from build123d import *

# Parameters (mm, degrees)
SKETCH002_W     = 13
SKETCH002_H     = 14
SKETCH002_W_2   = 6
PAD001_DEPTH    = 2
SKETCH_R        = 1.6
PAD_DEPTH       = 5
POCKET_DEPTH    = 10.001
SKETCH003_W     = 7
SKETCH003_H     = 5
POCKET001_DEPTH = 17.2330508076
SKETCH004_R     = 1
POCKET002_DEPTH = 6
POCKET003_DEPTH = 3
FILLET_R        = 8
FILLET001_R     = 1
FILLET002_R     = 1


with BuildPart() as pad001:
    # Sketch002 → Pad001 (new body, symmetric)
    with BuildSketch(Plane.XY):
        with Locations((-0.5, 0)):
            Rectangle(SKETCH002_W, SKETCH002_H)
        with Locations((-13, 0)):
            Rectangle(SKETCH002_W_2, SKETCH002_H)
    extrude(amount=PAD001_DEPTH, both=True)


with BuildPart() as fillet002:
    # Sketch → Pad (new body, symmetric)
    with BuildSketch(Plane.XY):
        with BuildLine():
            ThreePointArc((0, -4), (3.9731206567, -0.4629387079), (0.9196556715, 3.8928438764))
            Line((0.9196556715, 3.8928438764), (-8, 6))
            Line((-8, 6), (-30, 6))
            Line((-30, -4), (-30, 6))
            Line((0, -4), (-30, -4))
        make_face()
        Circle(SKETCH_R, mode=Mode.SUBTRACT)
    extrude(amount=PAD_DEPTH, both=True)

    # Sketch001 → Pocket (cut, through all)
    with BuildSketch(Plane(origin=(0, 6, 0), x_dir=(-1, 0, 0), z_dir=(0, 1, 0))):
        Polygon((22, 0.1132486541), (24, -3.3508529611), (24, -5), (30, -5), (30, 5), (27, 5), (27, 3), align=None)
    extrude(amount=-POCKET_DEPTH, mode=Mode.SUBTRACT)

    # Cut: cut Pad001
    add(pad001.part, mode=Mode.SUBTRACT)

    # Sketch003 → Pocket001 (cut, through all)
    with BuildSketch(Plane(origin=(-5.4509618943, 0, -9.4413429511), x_dir=(0.8660254038, 0, -0.5), z_dir=(-0.5, 0, -0.8660254038))):
        with Locations((-22.6091832103, -1)):
            Rectangle(SKETCH003_W, SKETCH003_H)
    extrude(amount=-POCKET001_DEPTH, mode=Mode.SUBTRACT)

    # Sketch004 → Pocket002 (cut)
    with BuildSketch(Plane(origin=(-16.5490381057, 0, 9.5545916051), x_dir=(0, -1, 0), z_dir=(-0.8660254038, 0, 0.5))):
        with Locations((-1, -7.9019237886)):
            Circle(SKETCH004_R)
    extrude(amount=-POCKET002_DEPTH, mode=Mode.SUBTRACT)

    # Sketch005 → Pocket003 (cut)
    with BuildSketch(Plane.YZ.offset(-7)):
        with BuildLine():
            Line((0.5, 1), (2.5, 1))
            ThreePointArc((2.5, -1), (3.5, 0), (2.5, 1))
            Line((0.5, -1), (2.5, -1))
            ThreePointArc((0.5, 1), (-0.5, 0), (0.5, -1))
        make_face()
    extrude(amount=-POCKET003_DEPTH, mode=Mode.SUBTRACT)

    # Fillet
    fillet_edges = [fillet002.edges().sort_by_distance(p)[0] for p in [
        (-8, 6, 0),
    ]]
    fillet(fillet_edges, radius=FILLET_R)

    # Fillet001
    fillet001_edges = [fillet002.edges().sort_by_distance(p)[0] for p in [
        (-27, 4.75, 5),
        (-27, -2.75, 5),
    ]]
    fillet(fillet001_edges, radius=FILLET001_R)

    # Fillet002
    fillet002_edges = [fillet002.edges().sort_by_distance(p)[0] for p in [
        (-19.178633, 1, 5),
    ]]
    fillet(fillet002_edges, radius=FILLET002_R)


solid = fillet002.part
Could you check a few things on this model? Use its own coordinates, in mm. A direction names the side the tool comes from. Coordinates: 2 decimals unless noted, no trailing zeros. Order: outer loops, then holes, each group sorted by start corner. A loop starts at its lowest first (then second) coordinate and runs counter-clockwise, first axis right, second up. Notation, with made-up numbers: (85, 21.5) -> (108, 21.5) arc R21 ccw to (108, 25.5) -> close; hole circle Ø9 at (56.5, 9). An arc over 180 degrees is marked (long way). One line per item, written item: value. Start each with the question number.
1) If I drill on L1, parallel to Z at x = -0.5, y = -3.25; L2, parallel to X at y = 0, z = -4.35; L3, parallel to Y at x = -22, z = 3, over which ranges is the centre line in solid material (lowest first)? Write a range as [from, to].
2) I'm going to push flat-ended pins straight in: pin 1 (2 mm diameter, centred on y = 2.5, z = -0.5, fed in from -X); pin 2 (2 mm diameter, centred on y = 0.5, z = -0.5, fed in from +X); pin 3 (5 mm diameter, centred on y = 2, z = -1, fed in from -X). Where does each tip first touch, or does it pass through?
3) Imagine slicing it at D-D on y = -2. List the corners of the cut face in (x, z) for me.
4) We'd pull the mould along X, two halves only. Please class faces 1 (the flat face through (-13, 1, 2)), 2 (the flat face through (-3.031, 4.826, 2.292)), 3 (the flat face through (-13.3, -4, 2.3)): +X half, -X half, draft (parallel to the pull), parting line (faces both ways), or undercut.
5) Imagine slicing it at C-C on x = -4.5. List the corners of the cut face in (y, z) for me, plus the area to 3 significant figures.
6) Imagine slicing it at B-B on x = -8. List the corners of the cut face in (y, z) for me, plus the area to 3 significant figures.
7) Imagine slicing it at A-A on z = -4. List the corners of the cut face in (x, y) for me, plus the area to 3 significant figures.
8) Which directions (+Z, -Z, +X, -X, +Y, -Y) give clear straight access to the entire face, cutting with the end or side of a thin tool? Please do faces 4 (the flat face through (-3, 1, 2)), 5 (the flat face through (-24, 1, -4)), 6 (the cylindrical face through (-8.5, -0.5, 0)), 7 (the flat face through (-24.535, -2.732, 1.577)), 8 (the flat face through (-10, 0.9, 1.4)).
Answer list:
1. L1: z = [-5, -2], [2, 5]
1. L2: x = [-24, -1.6], [1.6, 4]
1. L3: y = [-4, -1.5], [3.5, 6]
2. pin 1: stops at x = -22.93
2. pin 2: stops at x = -7
2. pin 3: stops at x = -24
3. outline: (-27, 3) -> (-22, 0.11) -> (-24, -3.35) -> (-24, -5) -> (3.46, -5) -> (3.46, -2) -> (-7, -2) -> (-7, 2) -> (3.46, 2) -> (3.46, 5) -> (-26, 5) arc R1 ccw to (-27, 4) -> close; hole (-16, -2) -> (-10, -2) -> (-10, 2) -> (-16, 2) -> close
4. face 1: undercut
4. face 2: +X half
4. face 3: draft
5. outline: (-4, -5) -> (5.17, -5) -> (5.17, -2) -> (-4, -2) -> close; (-4, 2) -> (5.17, 2) -> (5.17, 5) -> (-4, 5) -> close
5. area: 55.0 mm2
6. outline: (-4, -5) -> (5.95, -5) -> (5.95, 5) -> (-4, 5) -> close; hole (0.5, -1) -> (2.5, -1) arc R1 ccw to (2.5, 1) -> (0.5, 1) arc R1 ccw to start
6. area: 92.3 mm2
7. outline: (-24, -4) -> (0, -4) arc R4 ccw to (0.92, 3.89) -> (-7.09, 5.79) arc R8 ccw to (-8.93, 6) -> (-24, 6) -> close; hole circle Ø3.2 at (0, 0)
7. area: 250 mm2
8. face 4: +X, +Y, -Y
8. face 5: -Z, -X, +Y, -Y
8. face 6: +X
8. face 7: -X, +Y, -Y
8. face 8: +Y, -Y
